```python
from build123d import *

# Parameters (mm, degrees)
SKETCH1_R                    = 19.05
BOSS_EXTRUDE1_DEPTH          = 342.9
SKETCH2_R                    = 12.7
CUT_EXTRUDE1_DEPTH           = 343.9
F_1_1_4_7_TAPPED_HOLE1_D     = 28.17876
F_1_1_4_7_TAPPED_HOLE1_DEPTH = 49.022
F_1_1_4_7_TAPPED_HOLE1_TIP   = 8.465753589
F_1_1_4_7_TAPPED_HOLE2_D     = 28.17876
F_1_1_4_7_TAPPED_HOLE2_DEPTH = 49.022
F_1_1_4_7_TAPPED_HOLE2_TIP   = 8.465753589


with BuildPart() as part:
    # Sketch1 → Boss-Extrude1 (new body)
    with BuildSketch(Plane(origin=(0, 0, 0), x_dir=(1, 0, 0), z_dir=(0, 1, 0))):
        Circle(SKETCH1_R)
    extrude(amount=BOSS_EXTRUDE1_DEPTH)

    # Sketch2 → Cut-Extrude1 (cut, through all)
    with BuildSketch(Plane(origin=(0, 342.9, 0), x_dir=(1, 0, 0), z_dir=(0, 1, 0))):
        Circle(SKETCH2_R)
    extrude(amount=-CUT_EXTRUDE1_DEPTH, mode=Mode.SUBTRACT)

    # 1-1/4-7 Tapped Hole1
    with Locations(Plane(origin=(0, 342.9, 0), x_dir=(1, 0, 0), z_dir=(0, 1, 0))):
        with Locations((0, 0)):
            Hole(F_1_1_4_7_TAPPED_HOLE1_D / 2, depth=F_1_1_4_7_TAPPED_HOLE1_DEPTH)
            with Locations((0, 0, -(F_1_1_4_7_TAPPED_HOLE1_DEPTH + F_1_1_4_7_TAPPED_HOLE1_TIP / 2))):  # 118° drill point
                Cone(0, F_1_1_4_7_TAPPED_HOLE1_D / 2, F_1_1_4_7_TAPPED_HOLE1_TIP, mode=Mode.SUBTRACT)

    # 1-1/4-7 Tapped Hole2
    with Locations(Plane(origin=(0, 0, 0), x_dir=(-1, 0, 0), z_dir=(0, -1, 0))):
        with Locations((0, 0)):
            Hole(F_1_1_4_7_TAPPED_HOLE2_D / 2, depth=F_1_1_4_7_TAPPED_HOLE2_DEPTH)
            with Locations((0, 0, -(F_1_1_4_7_TAPPED_HOLE2_DEPTH + F_1_1_4_7_TAPPED_HOLE2_TIP / 2))):  # 118° drill point
                Cone(0, F_1_1_4_7_TAPPED_HOLE2_D / 2, F_1_1_4_7_TAPPED_HOLE2_TIP, mode=Mode.SUBTRACT)


solid = part.part
```
Build history of the part. All positions in model axes, mm. A direction names the side the tool comes from. Give positions to 0.01 mm unless a question says otherwise; leave off trailing zeros. Loops run counter-clockwise (first coordinate to the right, second up) from the corner with the lowest first, then second, coordinate; pieces in that order, holes last.
1) Two-plate mould, pull along Z, no slides. Class faces 1 (the face through (13.44, 24.85, -4.23)), 2 (the face through (-7, 0, 13)), 3 (the face through (-15.12, 169.05, 11.59)): released by +Z, released by -Z, zero draft, split by the parting line, or undercut.
Values follow:
face 1: undercut
face 2: zero draft
face 3: split by the parting line
2) Band-saw the part on C-C on y = 313. List the corners of the cut face in (x, z).
Values follow:
outline: circle Ø38.1 at (0, 0); hole circle Ø28.18 at (0, 0)
3) 3-axis set-ups, long thin cutter, end or side, ignore diameter. For faces 4 (the face through (-7, 342.9, 13)), 5 (the face through (-13.44, 318.05, -4.23)): which of +Z, -Z, +X, -X, +Y, -Y reach the whole face in a straight line?
Values follow:
face 4: +Z, -Z, +X, -X, +Y
face 5: +Y
4) Band-saw the part on D-D on y = 158.5. List the corners of the cut face in (x, z).
Values follow:
outline: circle Ø38.1 at (0, 0); hole circle Ø25.4 at (0, 0)
5) Band-saw the part on B-B on z = 0. List the corners of the cut face in (x, y), then the cut area to 3 significant figures.
Values follow:
outline: (-19.05, 0) - (-14.09, 0) - (-14.09, 49.02) - (-12.7, 49.86) - (-12.7, 293.04) - (-14.09, 293.88) - (-14.09, 342.9) - (-19.05, 342.9) - close; (12.7, 49.86) - (14.09, 49.02) - (14.09, 0) - (19.05, 0) - (19.05, 342.9) - (14.09, 342.9) - (14.09, 293.88) - (12.7, 293.04) - close
area: 4,080 mm2
6) Drop flat-ended pins along their axis: P1, Ø2, axis at x = -15, y = 151, coming from the -Z side; P2, Ø2, axis at y = 274, z = 11, coming from the +X side; P3, Ø4, axis at x = 6.5, y = 232.5, coming from the -Z side. Give the stop position or say it passes through.
Values follow:
P1: stops at z = -12.92
P2: stops at x = 16.21
P3: stops at z = -18.51
7) Band-saw the part on A-A on x = 0. List the corners of the cut face in (y, z), then the cut area to 3 significant figures.
Values follow:
outline: (0, -19.05) - (342.9, -19.05) - (342.9, -14.09) - (293.88, -14.09) - (293.04, -12.7) - (49.86, -12.7) - (49.02, -14.09) - (0, -14.09) - close; (0, 14.09) - (49.02, 14.09) - (49.86, 12.7) - (293.04, 12.7) - (293.88, 14.09) - (342.9, 14.09) - (342.9, 19.05) - (0, 19.05) - close
area: 4,080 mm2
8) Probe line 1 along Z through (x, y) = (0, 309.5); line 2 along Z through (x, y) = (0, 134). List the from-to ranges inside material, lowest first.
Values follow:
line 1: z = -19.05 to -14.09, 14.09 to 19.05
line 2: z = -19.05 to -12.7, 12.7 to 19.05
